Design review of the part built by this model. Coordinates are the model's own, in mm. Face numbers are marked on the shaded views. A direction names the side the tool comes from. Give positions to 0.01 mm unless a question says otherwise; leave off trailing zeros. Write each loop counter-clockwise with the first axis right and the second up, starting at its lowest first coordinate (ties: lowest second). Pieces come first, ordered by that corner, then holes. Notation, with made-up numbers: M 48.25,72 L 71.25,72 A20 cw 71.25,80 Z; hole C 37.5,58 d5. An arc over 180 degrees is marked long. Use a Markdown table: item, result. Add a question column.
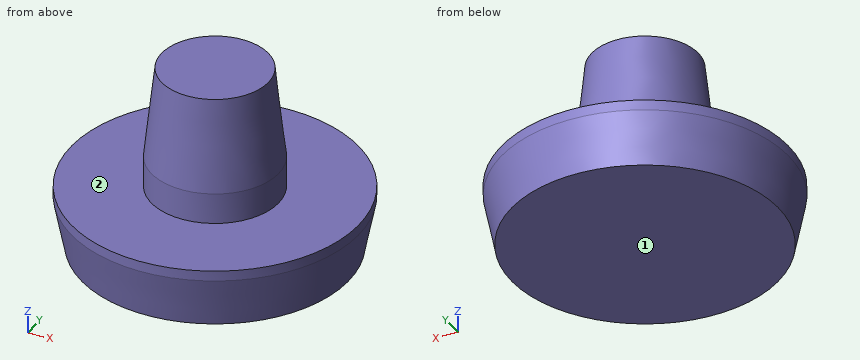
```python
from build123d import *

# Parameters (mm, degrees)
F0_R     = 7
F1_DEPTH = 3
F2_R     = 3.1
F3_DEPTH = 6
F4_SIZE2 = 4.5
F4_SIZE  = 0.5
F5_SIZE2 = 0.5
F5_SIZE  = 2.5


with BuildPart() as f1:
    # F0 (on Top) → F1 (new body)
    with BuildSketch(Plane.XY):
        Circle(F0_R)
    extrude(amount=F1_DEPTH)

    # F2 (on face) → F3 (join)
    with BuildSketch(Plane.XY.offset(3)):
        Circle(F2_R)
    extrude(amount=F3_DEPTH)

    # F4
    f4_edges = [f1.edges().sort_by_distance(p)[0] for p in [
        (-3.1, 0, 9),
    ]]
    f4_side = f1.faces().sort_by_distance((0, 0, 9))[0]
    chamfer(f4_edges, length=F4_SIZE, length2=F4_SIZE2, reference=f4_side)

    # F5
    f5_edges = [f1.edges().sort_by_distance(p)[0] for p in [
        (-7, 0, 0),
    ]]
    f5_side = f1.faces().sort_by_distance((-7, 0, 1.5))[0]
    chamfer(f5_edges, length=F5_SIZE, length2=F5_SIZE2, reference=f5_side)


solid = f1.part
```
(1) Wall thickness on L1, parallel to Z at x = -4.5, y = -4.25; L2, parallel to Y at x = 1.75, z = 0.75; L3, parallel to X at y = -0.75, z = 6.75: over which ranges is each line inside the solid? List them lowest first.
(2) Add section A-A on x = 0. Give the boundary of the cut face in (y, z).
(3) Add section C-C on z = 4. Give the boundary of the cut face in (x, y).
(4) For pin 1 (2 mm diameter, centred on x = 1.5, z = 1, fed in from -Y); pin 2 (2 mm diameter, centred on y = 1.5, z = 1, fed in from +X), all flat-tipped, find the tip position at first contact; note any pin that passes through.
(5) Add section D-D on z = 2. Give the boundary of the cut face in (x, y).
(6) Machinability: for the marked faces 1 and 2, which of the approach directions +Z, -Z, +X, -X, +Y, -Y give a long, thin tool a straight path to every point of the face, cutting with its end or side? Answer none if there is none.
From the geometry:
| question | item | result |
|---|---|---|
| 1 | L1 | z = 0 to 3 |
| 1 | L2 | y = -6.42 to 6.42 |
| 1 | L3 | x = -2.75 to 2.75 |
| 2 | outline | M -7,2.5 L -6.5,0 L 6.5,0 L 7,2.5 L 7,3 L 3.1,3 L 3.1,4.5 L 2.6,9 L -2.6,9 L -3.1,4.5 L -3.1,3 L -7,3 Z |
| 3 | outline | C 0,0 d6.2 |
| 4 | pin 1 | stops at y = -6.8 |
| 4 | pin 2 | stops at x = 6.8 |
| 5 | outline | C 0,0 d13.8 |
| 6 | face 1 | -Z, +X, -X, +Y, -Y |
| 6 | face 2 | +Z |
